Part model, mm, in its own coordinate system. A direction names the side the tool comes from. Round coordinates to 2 decimals unless told otherwise and drop trailing zeros. Order: outer loops, then holes, each group sorted by start corner. A loop starts at its lowest first (then second) coordinate and runs counter-clockwise, first axis right, second up. Notation, with made-up numbers: M -2.75,3.25 L 6.25,3.25 A27 ccw 6.25,34.25 Z; hole C 36.25,-39 d7. An arc over 180 degrees is marked long. Write each question's results on one line, items separated by ' | '. Start each with the question number.
1. Which spindle directions (+Z, -Z, +X, -X, +Y, -Y) get a long thin tool onto all of the face, cutting with end or side? Do faces 1 (the face through (130, -30, 43.245)), 2 (the face through (79, -19, 0)), 3 (the face through (130, -59, 96.365)). Say none if no direction does.
2. Two-plate mould, pull along X, no slides. Class faces 4 (the face through (19, 0, -1)), 5 (the face through (0, -19, 21)), 6 (the face through (0, -15, 97)), 7 (the face through (148.51, -18.78, 21.51)): +X half, -X half, draft (parallel to the pull), parting line (faces both ways), or undercut.
3. Probe L1, parallel to X at y = -70, z = 53.5; L2, parallel to Z at x = 187.5, y = -48.5; L3, parallel to X at y = -6, z = 27. List the from-to ranges inside material, lowest first. Write a range as [from, to].
4. Band-saw the part on D-D, the plane x = 183. List the corners of the cut face in (y, z), then the cut area to 3 significant figures.
5. Band-saw the part on A-A, the plane x = 64. List the corners of the cut face in (y, z).
6. Drop flat-ended pins along their axis: pin 1 Ø4 at (x, z) = (-12, -17.5) entering from +Y; pin 2 Ø12 at (y, z) = (23.5, 54.5) entering from -X; pin 3 Ø2 at (x, z) = (156, 64) entering from +Y. Give the stop position or say it passes through.
7. Band-saw the part on B-B, the plane z = 15.5. List the corners of the cut face in (x, y), then the cut area to 3 significant figures.
8. Band-saw the part on C-C, the plane y = -71.5. List the corners of the cut face in (x, z), then the cut area to 3 significant figures.
```python
from build123d import *

# Parameters (mm, degrees)
F1_DEPTH = 38.1
F3_DEPTH = 264.16


with BuildPart() as f1:
    # F0 (on Front) → F1 (new body)
    with BuildSketch(Plane.XZ):
        with BuildLine():
            Line((0, 101.651832), (-151.931614, 101.651832))
            Line((-151.931614, 101.651832), (0, -34.334853))
            Line((0, -34.334853), (155.22711, -34.334853))
            ThreePointArc((155.22711, -34.334853), (191.708041, 4.217474), (244.616956, 0))
            ThreePointArc((244.616956, 0), (199.922033, 77.341867), (155.22711, 0))
            Line((155.22711, 0), (0, 0))
            Line((0, 0), (0, 101.651832))
        make_face()
    extrude(amount=F1_DEPTH)

    # F2 (on Right) → F3 (join)
    with BuildSketch(Plane.YZ):
        Polygon((-14.352266, 96.364982), (-104.755044, 96.364982), (-104.755044, 43.245103), (46.02623, 43.245103), align=None)
    extrude(amount=F3_DEPTH)


solid = f1.part
```
Solution:
1) face 1: none | face 2: +Y, -Y | face 3: +Z, +X, +Y, -Y
2) face 4: draft | face 5: undercut | face 6: +X half | face 7: undercut
3) L1: [0, 264.16] | L2: [43.25, 96.36] | L3: [-68.53, 0], [148.35, 251.49]
4) outline: M -104.76,43.25 L -38.1,43.25 L -38.1,0.06 L 0,0.06 L 0,43.25 L 46.03,43.25 L -14.35,96.36 L -104.76,96.36 Z | area: 8,050 mm^2
5) outline: M -104.76,43.25 L 46.03,43.25 L -14.35,96.36 L -104.76,96.36 Z; M -38.1,-34.33 L 0,-34.33 L 0,0 L -38.1,0 Z
6) pin 1: y = 0 | pin 2: x = 0 | pin 3: y = 23.57
7) outline: M -55.68,-38.1 L 0,-38.1 L 0,0 L -55.68,0 Z; M 149.37,-38.1 L 250.48,-38.1 L 250.48,0 L 149.37,0 Z | area: 5,970 mm^2
8) outline: M 0,43.25 L 264.16,43.25 L 264.16,96.36 L 0,96.36 Z | area: 14,000 mm^2
